```python
from build123d import *

# Parameters (mm, degrees)
F0_R            = 12.7
F1_DEPTH        = 4.7625
F2_R            = 7.6
F3_DEPTH        = 4.7625
F4_R            = 9.45
F4_R_2          = 7.6
F5_DEPTH        = 19.8
F6_SIZE         = 0.2
F7_R            = 1.9
F9_DEPTH        = 4.7625
F9_COPIES_COUNT = 4
F10_R           = 3.0655
F11_DEPTH       = 29.325


# Not quite as in the source:
# - a pattern or mirror of a feature is missing from the dataset's text; its kind, count and spacing are read off the source's solid


with BuildPart() as f1:
    # F0 (on Front) → F1 (new body)
    with BuildSketch(Plane.XZ):
        Circle(F0_R)
    extrude(amount=F1_DEPTH)

    # F2 (on face) → F3 (join)
    with BuildSketch(Plane.XZ.offset(4.7625)):
        Circle(F2_R)
    extrude(amount=F3_DEPTH)

    # F4 (on face) → F5 (join)
    with BuildSketch(Plane.XZ.offset(9.525)):
        Circle(F4_R)
        Circle(F4_R_2, mode=Mode.SUBTRACT)
        Circle(F4_R_2)
    extrude(amount=F5_DEPTH)

    # F6
    f6_edges = [f1.edges().sort_by_distance(p)[0] for p in [
        (-12.7, 0, 0),
        (-12.7, -4.7625, 0),
    ]]
    chamfer(f6_edges, length=F6_SIZE)

    # F7 (on face) → F9 (cut, through all)
    with BuildSketch(Plane(origin=(0, 0, 0), x_dir=(-1, 0, 0), z_dir=(0, 1, 0))):
        with Locations((0, 9.6)):
            Circle(F7_R)
    f9 = extrude(amount=-F9_DEPTH, mode=Mode.SUBTRACT)

    # F9_copies: F9 ×4 about axis
    f9_copies_axis = Axis((0, 0, 0), (0, 1, 0))
    for i in range(1, F9_COPIES_COUNT):
        add(f9.rotate(f9_copies_axis, i * 360 / F9_COPIES_COUNT), mode=Mode.SUBTRACT)

    # F10 (on face) → F11 (cut, through all)
    with BuildSketch(Plane(origin=(0, 0, 0), x_dir=(-1, 0, 0), z_dir=(0, 1, 0))):
        Circle(F10_R)
    extrude(amount=-F11_DEPTH, mode=Mode.SUBTRACT)


solid = f1.part
```
Input: part model. Units: mm. Frame: model coordinates. A direction names the side the tool comes from. Coordinates: 2 decimals unless noted, no trailing zeros. Loops run counter-clockwise (first coordinate to the right, second up) from the corner with the lowest first, then second, coordinate; pieces in that order, holes last. Notation, with made-up numbers: M 79,51.25 L 89,51.25 A32 cw 89,86.25 Z; hole C -28,79.25 d5. An arc over 180 degrees is marked long. Use a Markdown table: item, result. Add a question column.
1) Pin query (flat end, axial travel): P1, Ø6, axis at y = -5.5, z = 5.5, coming from the -X side; P2, Ø1.5, axis at x = -7.5, y = -11.5, coming from the -Z side; P3, Ø2, axis at x = 3.5, y = -21.5, coming from the +Z side. Return the tip coordinate at first contact, or that it passes through.
2) Line query: L1, parallel to Z at x = 0, y = -17.75; L2, parallel to Y at x = 7, z = 4.5 (1 decimal); L3, parallel to Y at x = 11, z = 3.25. Output: solid intervals per line, ascending. Write a range as from..to.
3) Set-up query: faces 4 (the cylindrical face through (-0.247, -2.348, -11.484)), 5 (the flat face through (3, 0, -3)), 6 (the cylindrical face through (-7.593, -7.11, 0.334)), 7 (the cylindrical face through (9.014, -19.286, 2.839)). Return all of +Z, -Z, +X, -X, +Y, -Y with unobstructed straight access to the full face (end or side cutting, diameter ignored); none if empty.
4) Section B-B, the plane y = -3.5. Return the cut outline in (x, z).
5) Section A-A, the plane z = 0. Give the number of separate pieces and of enclosed holes in the cut face, plus the area to 3 significant figures.
6) Section D-D, the plane y = -27. Return the cut outline in (x, z).
7) Draft query along Z for faces 1 (the flat face through (4, -29.325, 0)), 2 (the cylindrical face through (-2.75, -2.35, -12.4)), 3 (the cylindrical face through (-11.484, -2.348, 0.247)). Return one class per face: +Z half, -Z half, draft (parallel to the pull), parting line (faces both ways), or undercut.
Answer below:
| question | item | result |
|---|---|---|
| 1 | P1 | x = -12.42 |
| 1 | P2 | z = -6.61 |
| 1 | P3 | z = 9.11 |
| 2 | L1 | -9.45..-3.07, 3.07..9.45 |
| 2 | L2 | -29.3..-9.5, -4.8..0 |
| 2 | L3 | -4.76..0 |
| 3 | face 4 | +Y |
| 3 | face 5 | +Z, -Z, +X, -X, +Y |
| 3 | face 6 | none |
| 3 | face 7 | -Y |
| 4 | outline | C 0,0 d25.4; hole C -9.6,0 d3.8; hole C 0,0 d6.13; hole C 0,-9.6 d3.8; hole C 0,9.6 d3.8; hole C 9.6,0 d3.8 |
| 5 | separate pieces | 4 |
| 5 | enclosed holes | 0 |
| 5 | area | 352 mm2 |
| 6 | outline | C 0,0 d18.9; hole C 0,0 d6.13 |
| 7 | face 1 | draft |
| 7 | face 2 | parting line |
| 7 | face 3 | undercut |
